For this review, take the finished solid that the model builds, in its own axes (mm). A direction names the side the tool comes from. Coordinates: 2 decimals unless noted, no trailing zeros. Order: outer loops, then holes, each group sorted by start corner. A loop starts at its lowest first (then second) coordinate and runs counter-clockwise, first axis right, second up. Notation, with made-up numbers: (-7, 42.5) -> (20, 42.5) arc R30 cw to (20, 77.5) -> close; hole circle Ø2 at (37.5, 28). An arc over 180 degrees is marked (long way). Write item = value, one per line. Start each with the question number.
1) Machinability: for faces 4 (the face through (-2.76, 19.43, 0.51)), 5 (the face through (41.64, 26.1, 0.51)), 6 (the face through (-23.12, 22.7, 0.51)), which of the approach directions +Z, -Z, +X, -X, +Y, -Y give a long, thin tool a straight path to every point of the face, cutting with its end or side? Answer none if there is none.
2) Consider section B-B on y = 22. Give the boundary of the cut face in (x, z), and give its area (3 significant figures).
3) Consider section C-C on x = 13.5. Give the boundary of the cut face in (y, z).
4) Draft analysis for pull direction X (two halves, no side actions). For faces 1 (the face through (2.76, 22.57, 0.51)), 2 (the face through (28.474, 9.302, 0.507)), 3 (the face through (-1, 0, 0)), state which applies: +X half, -X half, draft (parallel to the pull), parting line (faces both ways), or undercut.
5) Consider section D-D on z = 0.2. State how many separate pieces and enclosed holes the cut face has, and give its area (3 significant figures).
6) Consider section A-A on x = -12. Give the boundary of the cut face in (y, z).
7) Wall thickness on probe 1 along X at (y, z) = (19, 0.2); probe 2 along Y at (x, z) = (-30.5, 0.15); probe 3 along X at (y, z) = (22, 0.85): over which ranges is each line inside the solid? List them lowest first. Write a range as [from, to].
from build123d import *

# Parameters (mm, degrees)
F0_W      = 85
F0_H      = 54
F1_DEPTH  = 1
F2_R      = 3
F4_DEPTH  = 1.001
F5_W      = 4
F5_H      = 3.55
F5_H_2    = 3.4
F5_H_3    = 3.3
F6_DEPTH  = 1.001
F8_DEPTH  = 1.001
F10_DEPTH = 1.001
F11_R     = 0.5
F13_DEPTH = 1.001


with BuildPart() as f1:
    # F0 (on Top) → F1 (new body)
    with BuildSketch(Plane.XY):
        Rectangle(F0_W, F0_H)
    extrude(amount=F1_DEPTH)

    # F2
    f2_edges = [f1.edges().sort_by_distance(p)[0] for p in [
        (-42.5, -27, 0.5),
        (-42.5, 27, 0.5),
        (42.5, -27, 0.5),
        (42.5, 27, 0.5),
    ]]
    fillet(f2_edges, radius=F2_R)

    # F3 (on face) → F4 (cut, through all)
    with BuildSketch(Plane.XY.offset(1)):
        Polygon((-22.5925227119, -3.5), (-32.4074772881, -3.5), (-37.3149545762, -12), (-32.4074772881, -20.5), (-22.5925227119, -20.5), (-13.932268674, -20.5), (-5.8493649054, -20.5), (1.6561885941, -20.5), (8.5843918244, -20.5), (14.3578945162, -20.5), (18.9766966698, -20.5), (21.2860977465, -16.5), (18.9766966698, -12.5), (15.5125950546, -12.5), (14.3578945162, -10.5), (9.7390923627, -10.5), (8.5843918244, -8.5), (2.2335388633, -8.5), (1.6561885941, -7.5), (-5.2720146362, -7.5), (-5.8493649054, -6.5), (-13.3549184049, -6.5), (-13.932268674, -5.5), (-21.4378221735, -5.5), align=None)
    extrude(amount=-F4_DEPTH, mode=Mode.SUBTRACT)

    # F5 (on face) → F6 (cut, through all)
    with BuildSketch(Plane.XY.offset(1)):
        with Locations((40.5, -7.525)):
            Rectangle(F5_W, F5_H)
        with Locations((40.5, -14)):
            Rectangle(F5_W, F5_H_2)
        with Locations((40.5, -20.35)):
            Rectangle(F5_W, F5_H_3)
    extrude(amount=-F6_DEPTH, mode=Mode.SUBTRACT)

    # F7 (on face) → F8 (cut, through all)
    with BuildSketch(Plane.XY.offset(1)):
        Polygon((42.5, 20.5), (30.6698729811, 20.5), (26.3397459622, 13), (30.6698729811, 5.5), (42.5, 5.5), align=None)
    extrude(amount=-F8_DEPTH, mode=Mode.SUBTRACT)

    # F9 (on face) → F10 (cut, through all)
    with BuildSketch(Plane.XY.offset(1)):
        with BuildLine():
            Line((-32.5, 27), (-32.5, 26))
            ThreePointArc((-32.5, 26), (-36.3687561178, 20.9837686773), (-30.5342244266, 18.5163630506))
            Line((-30.5342244266, 18.5163630506), (-15.5, 27))
            Line((-15.5, 27), (-32.5, 27))
        make_face()
    extrude(amount=-F10_DEPTH, mode=Mode.SUBTRACT)

    # F11
    f11_edges = [f1.edges().sort_by_distance(p)[0] for p in [
        (-32.5, 26, 0.5),
        (-32.5, 27, 0.5),
    ]]
    fillet(f11_edges, radius=F11_R)

    # F12 (on face) → F13 (cut, through all)
    with BuildSketch(Plane.XY.offset(1)):
        Polygon((1.8330871047, 24.175), (-1.8330871047, 24.175), (-3.6661742094, 21), (-1.8330871047, 17.825), (1.8330871047, 17.825), (3.6661742094, 21), align=None)
        Polygon((34.3330871047, -17.825), (30.6669128953, -17.825), (28.8338257906, -21), (30.6669128953, -24.175), (34.3330871047, -24.175), (36.1661742094, -21), align=None)
        Polygon((-34.6669128953, 10.175), (-38.3330871047, 10.175), (-40.1661742094, 7), (-38.3330871047, 3.825), (-34.6669128953, 3.825), (-32.8338257906, 7), align=None)
    extrude(amount=-F13_DEPTH, mode=Mode.SUBTRACT)


solid = f1.part
Answer sheet:
q1.face_4 = +Z, -Z
q1.face_5 = +Z, -Z, +X, +Y
q1.face_6 = +Z, -Z, +Y
q2.outline = (-42.5, 0) -> (-36.5, 0) -> (-36.5, 1) -> (-42.5, 1) -> close; (-24.36, 0) -> (-3.09, 0) -> (-3.09, 1) -> (-24.36, 1) -> close; (3.09, 0) -> (42.5, 0) -> (42.5, 1) -> (3.09, 1) -> close
q2.area = 66.7 mm2
q3.outline = (-27, 0) -> (-20.5, 0) -> (-20.5, 1) -> (-27, 1) -> close; (-10.5, 0) -> (27, 0) -> (27, 1) -> (-10.5, 1) -> close
q4.face_1 = undercut
q4.face_2 = +X half
q4.face_3 = draft
q5.separate_pieces = 1
q5.enclosed_holes = 4
q5.area = 3,380 mm2
q6.outline = (-27, 0) -> (-20.5, 0) -> (-20.5, 1) -> (-27, 1) -> close; (-6.5, 0) -> (27, 0) -> (27, 1) -> (-6.5, 1) -> close
q7.probe_1 = [-42.5, -35.15], [-29.68, -2.51], [2.51, 29.8]
q7.probe_2 = [-27, -20.5], [-3.5, 18.54]
q7.probe_3 = [-42.5, -36.5], [-24.36, -3.09], [3.09, 42.5]
